```python
from build123d import *

# Parameters (mm, degrees)
BOSS_EXTRUDE1_DEPTH = 10
SKETCH2_R           = 1.5
CUT_EXTRUDE1_DEPTH  = 2
SKETCH3_R           = 4
CUT_EXTRUDE2_DEPTH  = 2
FILLET1_R           = 1


with BuildPart() as part:
    # Sketch1 → Boss-Extrude1 (new body)
    with BuildSketch(Plane(origin=(0, 0, 0), x_dir=(1, 0, 0), z_dir=(0, 1, 0))):
        Polygon((12, 5), (12, -27.5), (2, -27.5), (2, -22.5), (0, -22.5), (0, -29.5), (12, -29.5), (12, -58), (14, -58), (14, 7), (0, 7), (0, 0), (2, 0), (2, 5), align=None)
    extrude(amount=BOSS_EXTRUDE1_DEPTH)

    # Sketch2 → Cut-Extrude1 (cut)
    with BuildSketch(Plane.ZY):
        with Locations((25.15, 5)):
            Circle(SKETCH2_R)
        with Locations((-2.65, 5)):
            Circle(SKETCH2_R)
    extrude(amount=-CUT_EXTRUDE1_DEPTH, mode=Mode.SUBTRACT)

    # Sketch3 → Cut-Extrude2 (cut)
    with BuildSketch(Plane.ZY.offset(-12)):
        with Locations((16.4, 5)):
            Circle(SKETCH3_R)
        with BuildLine():
            Line((50.197224362, 8), (53.802775638, 8))
            ThreePointArc((53.802775638, 8), (52, 1.5), (50.197224362, 8))
        make_face()
    extrude(amount=-CUT_EXTRUDE2_DEPTH, mode=Mode.SUBTRACT)

    # Fillet1
    fillet1_edges = [part.edges().sort_by_distance(p)[0] for p in [
        (2, 5, 27.5),
        (12, 5, 27.5),
        (12, 5, -5),
        (2, 5, -5),
        (0, 5, -7),
        (14, 5, -7),
        (12, 5, 29.5),
        (0, 5, 29.5),
    ]]
    fillet(fillet1_edges, radius=FILLET1_R)


solid = part.part
```
Part model, mm, in its own coordinate system. A direction names the side the tool comes from. Coordinates: 2 decimals unless noted, no trailing zeros. Order: outer loops, then holes, each group sorted by start corner. A loop starts at its lowest first (then second) coordinate and runs counter-clockwise, first axis right, second up. Notation, with made-up numbers: (71.25, -35.5) -> (130.25, -35.5) arc R7 cw to (130.25, -27.5) -> close; hole circle Ø9 at (-2, 71). An arc over 180 degrees is marked (long way). Put each result on its own line as item: value. Start each with the question number.
(1) Mould opens along Y. For faces 6 (the face through (0.99, 5.45, 26.58)), 7 (the face through (2, 5, 23)), 8 (the face through (13, 1.5, 52.1)), 9 (the face through (12.2, 0, 20.5)) say: pulls with the +Y half, pulls with the -Y half, needs draft (parallel to the pull), parting line crosses it, or undercut.
(2) Which spindle directions (+Z, -Z, +X, -X, +Y, -Y) get a long thin tool onto all of the face, cutting with end or side? Do faces 1 (the face through (12.2, 10, 20.5)), 2 (the face through (1, 5, 22.5)), 3 (the face through (6, 5, 29.5)), 4 (the face through (0.99, 5.45, -1.22)), 5 (the face through (12, 5, 11)). Say none if no direction does.
(3) Pin check, flat tips, straight feed: pin 1 Ø2.5 at (y, z) = (5, -2.65) entering from -X; pin 2 Ø2 at (x, y) = (0.5, 6) entering from +Z. Stop position of each tip, or through.
(4) Band-saw the part on A-A (z = 25.15). Give the cut face in (x, y), then the cut area to 3 significant figures.
(5) Band-saw the part on D-D (z = 4). Give the cut face in (x, y).
(6) Band-saw the part on C-C (z = 52). Give the cut face in (x, y), then the cut area to 3 significant figures.
(7) Probe line 1 along Z through (x, y) = (1.1, 5); line 2 along Y through (x, z) = (1.55, 25.15); line 3 along Z through (x, y) = (4.75, 2.5). List the from-to ranges inside material, lowest first. Write a range as [from, to].
(8) Band-saw the part on B-B (x = 5). Give the cut face in (y, z).
Determined:
1. face 6: undercut
1. face 7: needs draft
1. face 8: undercut
1. face 9: pulls with the -Y half
2. face 1: +Z, -Z, +X, -X, +Y
2. face 2: -X, +Y, -Y
2. face 3: +Z, -X, +Y, -Y
2. face 4: -X
2. face 5: +Y, -Y
3. pin 1: stops at x = 12
3. pin 2: stops at z = 29.5
4. outline: (0, 0) -> (2, 0) -> (2, 3.5) -> (0, 3.5) -> close; (0, 6.5) -> (2, 6.5) -> (2, 10) -> (0, 10) -> close; (12, 0) -> (14, 0) -> (14, 10) -> (12, 10) -> close
4. area: 34.0 mm²
5. outline: (12, 0) -> (14, 0) -> (14, 10) -> (12, 10) -> close
6. outline: (12, 0) -> (14, 0) -> (14, 1.5) -> (12, 1.5) -> close; (12, 8) -> (14, 8) -> (14, 10) -> (12, 10) -> close
6. area: 7.00 mm²
7. line 1: z = [-7, -4.15], [-1.15, 0], [22.5, 23.65], [26.65, 29.5]
7. line 2: y = [0, 3.5], [6.5, 10]
7. line 3: z = [-7, -5], [27.5, 29.5]
8. outline: (0, -7) -> (10, -7) -> (10, -5) -> (0, -5) -> close; (0, 27.5) -> (10, 27.5) -> (10, 29.5) -> (0, 29.5) -> close
